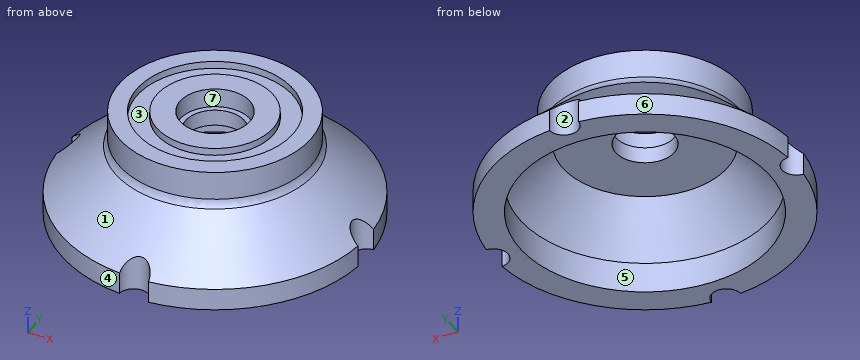
from build123d import *

# Parameters (mm, degrees)
CUT_EXTRUDE1_REACH = 34.929
SKETCH3_R          = 2
FILLET1_R          = 1.5


with BuildPart() as part:
    # Sketch2 → Revolve1 (revolve)
    with BuildSketch(Plane(origin=(0, 0, 0), x_dir=(0, 0, -1), z_dir=(1, 0, 0))):
        Polygon((0, 17), (0, 20.8), (-3, 20.8), (-10.2, 13), (-14.8, 13), (-14.8, 10.6), (-13.8, 10.6), (-13.8, 7.9), (-14.8, 7.9), (-14.8, 4.75), (-12.2, 4.75), (-12.2, 4), (-10, 4), (-10, 11.2), (-4.2, 17), align=None)
    revolve(axis=Axis((0, 0, 0), (0, 0, 1)))

    # Cut-Extrude1: up to this cone (the profile starts inside it)
    cut_extrude1_end = Plane(origin=(0, 0, 0), z_dir=(0, 0, -1)).offset(-22.199999) * Cone(1.083e-06, 88.485583333, 81.678999, align=(Align.CENTER, Align.CENTER, Align.MIN), mode=Mode.PRIVATE)
    # Sketch3 → Cut-Extrude1 (cut, up to the surface)
    with BuildSketch(Plane.XY, mode=Mode.PRIVATE) as cut_extrude1_sk1:
        with Locations((0, 20.8)):
            Circle(SKETCH3_R)
    cut_extrude1_tool1 = extrude(cut_extrude1_sk1.sketch, amount=CUT_EXTRUDE1_REACH, mode=Mode.PRIVATE) & cut_extrude1_end
    add(cut_extrude1_tool1.solids().sort_by_distance((0, 20.8, 0))[0], mode=Mode.SUBTRACT)
    # Sketch3 → Cut-Extrude1 (cut, up to the surface)
    with BuildSketch(Plane.XY, mode=Mode.PRIVATE) as cut_extrude1_sk2:
        with Locations((20.8, 0)):
            Circle(SKETCH3_R)
    cut_extrude1_tool2 = extrude(cut_extrude1_sk2.sketch, amount=CUT_EXTRUDE1_REACH, mode=Mode.PRIVATE) & cut_extrude1_end
    add(cut_extrude1_tool2.solids().sort_by_distance((20.8, 0, 0))[0], mode=Mode.SUBTRACT)
    # Sketch3 → Cut-Extrude1 (cut, up to the surface)
    with BuildSketch(Plane.XY, mode=Mode.PRIVATE) as cut_extrude1_sk3:
        with Locations((0, -20.8)):
            Circle(SKETCH3_R)
    cut_extrude1_tool3 = extrude(cut_extrude1_sk3.sketch, amount=CUT_EXTRUDE1_REACH, mode=Mode.PRIVATE) & cut_extrude1_end
    add(cut_extrude1_tool3.solids().sort_by_distance((0, -20.8, 0))[0], mode=Mode.SUBTRACT)
    # Sketch3 → Cut-Extrude1 (cut, up to the surface)
    with BuildSketch(Plane.XY, mode=Mode.PRIVATE) as cut_extrude1_sk4:
        with Locations((-20.8, 0)):
            Circle(SKETCH3_R)
    cut_extrude1_tool4 = extrude(cut_extrude1_sk4.sketch, amount=CUT_EXTRUDE1_REACH, mode=Mode.PRIVATE) & cut_extrude1_end
    add(cut_extrude1_tool4.solids().sort_by_distance((-20.8, 0, 0))[0], mode=Mode.SUBTRACT)

    # Fillet1
    fillet1_edges = [part.edges().sort_by_distance(p)[0] for p in [
        (0, -13, 10.2),
    ]]
    fillet(fillet1_edges, radius=FILLET1_R)


solid = part.part
Input: part model. Units: mm. Frame: model coordinates. Face numbers are marked on the shaded views. A direction names the side the tool comes from. Round coordinates to 2 decimals unless told otherwise and drop trailing zeros.
1. Material intervals for line 1 (Y direction, x = 0, z = 14.4); line 2 (X direction, y = 0, z = 10.8), sorted ascending.
The answers:
line 1: y = -13 to -10.6, -7.9 to -4.75, 4.75 to 7.9, 10.6 to 13
line 2: x = -13 to -4, 4 to 13
2. Mould query, pull axis Y, two halves, no side actions, for the marked faces 1, 2, 3 and 4. Classes: released by +Y, released by -Y, zero draft, split by the parting line, or undercut.
The answers:
face 1: split by the parting line
face 2: released by +Y
face 3: undercut
face 4: released by -Y
3. Pin query (flat end, axial travel): P1, Ø4, axis at x = -5.5, z = 8, coming from the -Y side; P2, Ø6, axis at x = 14.5, z = 2.5, coming from the -Y side; P3, Ø6.5, axis at x = 0, y = 0, coming from the +Z side; P4, Ø3, axis at x = 14, y = -12, coming from the +Z side. Return the tip coordinate at first contact, or that it passes through.
The answers:
P1: stops at y = -16.75
P2: stops at y = -17.33
P3: passes through
P4: stops at z = 6.56
4. Set-up query: the marked faces 5, 6 and 7. Return all of +Z, -Z, +X, -X, +Y, -Y with unobstructed straight access to the full face (end or side cutting, diameter ignored); none if empty.
The answers:
face 5: -Z
face 6: +Z, -Z, -X, +Y
face 7: +Z
